```python
from build123d import *

# Parameters (mm, degrees)
SKETCH_1_R          = 8
EXTRUDE_1_DEPTH     = 2.5
SKETCH_2_R          = 2.5
CUT_EXTRUDE_1_DEPTH = 6
SKETCH_3_R          = 6.65
SKETCH_3_R_2        = 4.2
CUT_EXTRUDE_2_DEPTH = 0.5


with BuildPart() as part:
    # 草圖1 → 填料-伸長1 (new body, symmetric)
    with BuildSketch(Plane.XY):
        Circle(SKETCH_1_R)
    extrude(amount=EXTRUDE_1_DEPTH, both=True)

    # 草圖2 → 除料-伸長1 (cut, through all)
    with BuildSketch(Plane.XY.offset(2.5)):
        Circle(SKETCH_2_R)
    extrude(amount=-CUT_EXTRUDE_1_DEPTH, mode=Mode.SUBTRACT)

    # 草圖3 → 除料-伸長2 (cut)
    with BuildSketch(Plane.XY.offset(2.5)):
        Circle(SKETCH_3_R)
        Circle(SKETCH_3_R_2, mode=Mode.SUBTRACT)
    cut_extrude_2 = extrude(amount=-CUT_EXTRUDE_2_DEPTH, mode=Mode.SUBTRACT)

    # 鏡射1: 除料-伸長2 across plane
    add(cut_extrude_2.mirror(Plane.XY), mode=Mode.SUBTRACT)


solid = part.part
```
Design review of the part built by this model. Coordinates are the model's own, in mm. A direction names the side the tool comes from. Give positions to 0.01 mm unless a question says otherwise; leave off trailing zeros. Loops run counter-clockwise (first coordinate to the right, second up) from the corner with the lowest first, then second, coordinate; pieces in that order, holes last. Notation, with made-up numbers: M 27,44.5 L 63,44.5 A15 cw 63,61.5 Z; hole C -6.75,17 d4. An arc over 180 degrees is marked long. Return JSON: item names as keys, results as strings. Group by question number.
Item 1: We need section A-A (y = 0). Give the boundary of the cut face in (x, z).
Item 2: Mouldability with a two-part tool opening along Y and no side actions: class faces 4 (the flat face through (2, -2, -2.5)), 5 (the cylindrical face through (4.006, 1.262, -2.254)), 6 (the cylindrical face through (-1.73, -7.81, 0.04)) as released by +Y, released by -Y, zero draft, split by the parting line, or undercut.
Item 3: Insertion check: pin 1 Ø1 at (x, z) = (-2, 0.5) entering from -Y; pin 2 Ø2 at (y, z) = (3, 0) entering from -X; pin 3 Ø1 at (x, z) = (2, 1) entering from +Y. Each pin has a flat end and moves straight along its axis. Give the tip position at first contact, or say it passes through.
Item 4: For probe 1 along Y at (x, z) = (0, -2.35); probe 2 along Y at (x, z) = (0, -0.55); probe 3 along Y at (x, z) = (1, -2.2), list the stretches that pass through material, from the lowest coordinate up.
Item 5: Tool access review of faces 1 (the flat face through (4.3, -1.4, 2)), 2 (the flat face through (1, 7, -2.5)), 3 (the flat face through (4.3, -1.4, -2)): name each direction out of +Z, -Z, +X, -X, +Y, -Y from which nothing blocks a thin tool from reaching the whole face with its end or side.
Item 6: We need section D-D (y = -3). Give the boundary of the cut face in (x, z), and give its area (3 significant figures).
Item 7: We need section C-C (z = -1). Give the boundary of the cut face in (x, y), and give its area (3 significant figures).
Output:
{
 "1": {"outline": "M -8,-2.5 L -6.65,-2.5 L -6.65,-2 L -4.2,-2 L -4.2,-2.5 L -2.5,-2.5 L -2.5,2.5 L -4.2,2.5 L -4.2,2 L -6.65,2 L -6.65,2.5 L -8,2.5 Z; M 2.5,-2.5 L 4.2,-2.5 L 4.2,-2 L 6.65,-2 L 6.65,-2.5 L 8,-2.5 L 8,2.5 L 6.65,2.5 L 6.65,2 L 4.2,2 L 4.2,2.5 L 2.5,2.5 Z"},
 "2": {"face 4": "zero draft", "face 5": "undercut", "face 6": "split by the parting line"},
 "3": {"pin 1": "stops at y = -7.86", "pin 2": "stops at x = -7.75", "pin 3": "stops at y = 7.86"},
 "4": {"probe 1": "y = -8 to -6.65, -4.2 to -2.5, 2.5 to 4.2, 6.65 to 8", "probe 2": "y = -8 to -2.5, 2.5 to 8", "probe 3": "y = -7.94 to -6.57, -4.08 to -2.29, 2.29 to 4.08, 6.57 to 7.94"},
 "5": {"face 1": "+Z", "face 2": "-Z, +X, -X, +Y, -Y", "face 3": "-Z"},
 "6": {"outline": "M -7.42,-2.5 L -5.93,-2.5 L -5.93,-2 L -2.94,-2 L -2.94,-2.5 L 2.94,-2.5 L 2.94,-2 L 5.93,-2 L 5.93,-2.5 L 7.42,-2.5 L 7.42,2.5 L 5.93,2.5 L 5.93,2 L 2.94,2 L 2.94,2.5 L -2.94,2.5 L -2.94,2 L -5.93,2 L -5.93,2.5 L -7.42,2.5 Z", "area": "68.2 mm^2"},
 "7": {"outline": "C 0,0 d16; hole C 0,0 d5", "area": "181 mm^2"}
}
